from build123d import *

# Parameters (mm, degrees)
SKETCH1_R           = 19.5
BOSS_EXTRUDE1_DEPTH = 35.433
SKETCH2_R           = 9.9822
BOSS_EXTRUDE2_DEPTH = 4.953
SKETCH4_R           = 3
BOSS_EXTRUDE3_DEPTH = 11.7856
SKETCH5_R           = 1.58
CUT_EXTRUDE1_DEPTH  = 5.08


with BuildPart() as part:
    # Sketch1 → Boss-Extrude1 (new body)
    with BuildSketch(Plane.XY):
        Circle(SKETCH1_R)
    extrude(amount=-BOSS_EXTRUDE1_DEPTH)

    # Sketch2 → Boss-Extrude2 (add)
    with BuildSketch(Plane.XY):
        Circle(SKETCH2_R)
    extrude(amount=BOSS_EXTRUDE2_DEPTH)

    # Sketch4 → Boss-Extrude3 (add)
    with BuildSketch(Plane.XY.offset(4.953)):
        Circle(SKETCH4_R)
    extrude(amount=BOSS_EXTRUDE3_DEPTH)

    # Sketch5 → Cut-Extrude1 (cut)
    with BuildSketch(Plane.XY):
        with Locations((-11.944395574, -6.8961)):
            Circle(SKETCH5_R)
        with Locations((11.944395574, -6.8961)):
            Circle(SKETCH5_R)
        with Locations((0, 13.7922)):
            Circle(SKETCH5_R)
        with Locations((8.755768371, 12.253167763)):
            Circle(SKETCH5_R)
        with Locations((6.233670374, -13.709301721)):
            Circle(SKETCH5_R)
        with Locations((-14.989438745, 1.456133958)):
            Circle(SKETCH5_R)
    extrude(amount=-CUT_EXTRUDE1_DEPTH, mode=Mode.SUBTRACT)


solid = part.part
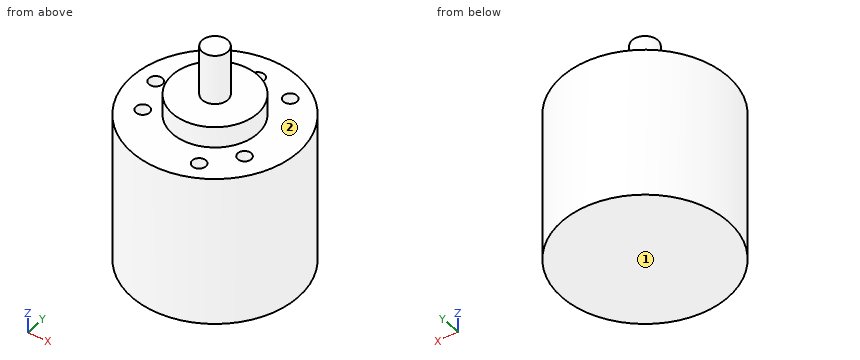
For this review, take the finished solid that the model builds, in its own axes (mm). Face numbers are marked on the shaded views. A direction names the side the tool comes from. Round coordinates to 2 decimals unless told otherwise and drop trailing zeros. Loops run counter-clockwise (first coordinate to the right, second up) from the corner with the lowest first, then second, coordinate; pieces in that order, holes last. Notation, with made-up numbers: (54, 82) - (99, 82) arc R28 ccw to (99, 117) - close; hole circle Ø3 at (14, 75). An arc over 180 degrees is marked (long way). Put each result on its own line as item: value. Start each with the question number.
1. Consider section C-C on z = -8.5. State the section outline as (x, y) points.
2. Insertion check: P1, Ø0.9, axis at x = 12, y = -7.5, coming from the +Z side; P2, Ø1.5, axis at y = 10.5, z = -25.5, coming from the +X side; P3, Ø2, axis at x = -4.5, y = -11, coming from the +Z side. Each pin has a flat end and moves straight along its axis. Give the tip position at first contact, or say it passes through.
3. For probe 1 along Y at (x, z) = (0, -2.65); probe 2 along Z at (x, y) = (-12, -14); probe 3 along Z at (x, y) = (3, -3.5), list the stretches that pass through material, from the lowest coordinate up. Write a range as [from, to].
4. For the marked faces 1 and 2, list the 3-axis set-ups (+Z, -Z, +X, -X, +Y, -Y) from which the entire face can be reached by the end or side of a thin tool; tool diameter is ignored.
5. Consider section B-B on z = -1. State the section outline as (x, y) points.
6. Consider section A-A on x = 0. State the section outline as (y, z) points.
7. Consider section D-D on x = -15.5. State the section outline as (y, z) points, plus the area to 3 significant figures.
Result sheet:
1. outline: circle Ø39 at (0, 0)
2. P1: z = -5.08
2. P2: x = 16.89
2. P3: z = 0
3. probe 1: [-19.5, 12.21], [15.37, 19.5]
3. probe 2: [-35.43, 0]
3. probe 3: [-35.43, 4.95]
4. face 1: -Z, +X, -X, +Y, -Y
4. face 2: +Z
5. outline: circle Ø39 at (0, 0); hole circle Ø3.16 at (-14.99, 1.46); hole circle Ø3.16 at (-11.94, -6.9); hole circle Ø3.16 at (0, 13.79); hole circle Ø3.16 at (6.23, -13.71); hole circle Ø3.16 at (8.76, 12.25); hole circle Ø3.16 at (11.94, -6.9)
6. outline: (-19.5, -35.43) - (19.5, -35.43) - (19.5, 0) - (15.37, 0) - (15.37, -5.08) - (12.21, -5.08) - (12.21, 0) - (9.98, 0) - (9.98, 4.95) - (3, 4.95) - (3, 16.74) - (-3, 16.74) - (-3, 4.95) - (-9.98, 4.95) - (-9.98, 0) - (-19.5, 0) - close
7. outline: (-11.83, -35.43) - (11.83, -35.43) - (11.83, 0) - (2.95, 0) - (2.95, -5.08) - (-0.04, -5.08) - (-0.04, 0) - (-11.83, 0) - close
7. area: 823 mm^2
